Study the drawing (mm; zero at the part's minimum x, y, z) and answer. A direction names the side the tool comes from. Coordinates: 2 decimals unless noted, no trailing zeros. Order: outer loops, then holes, each group sorted by start corner. A loop starts at its lowest first (then second) coordinate and runs counter-clockwise, first axis right, second up.
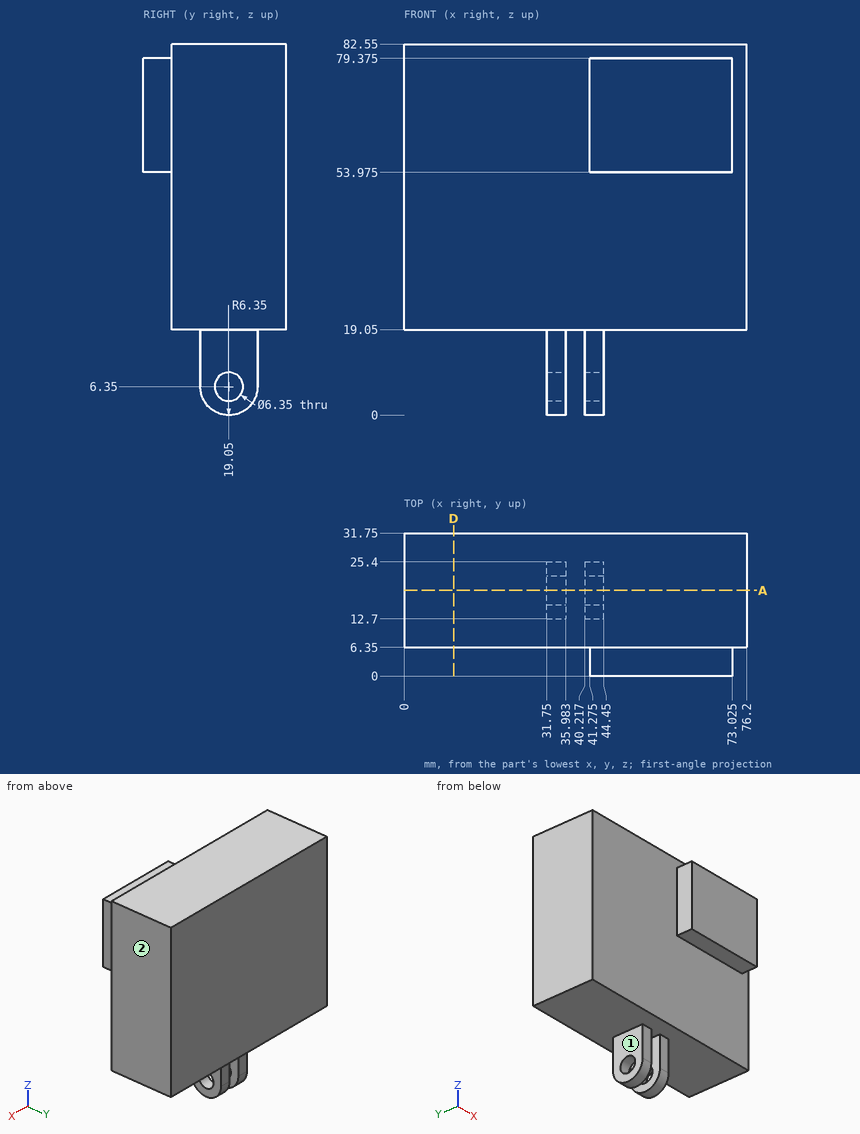
(1) Find section D-D (x = 11). Write down the section's boundary in (y, z).
(2) Each of these flat-tipped pins is pushed along its axis until it touches: pin 1 Ø8.5 at (y, z) = (19.05, 6.35) entering from +X; pin 2 Ø14 at (y, z) = (17, 6) entering from -X; pin 3 Ø3.5 at (x, z) = (33, 14) entering from +Y. Where does it stop, or does it pass through?
(3) Consider line 1 (Y direction, x = 41, z = 6) (1 decimal); line 2 (Y direction, x = 16.5, z = 30); line 3 (Z direction, x = 11.5, y = 11). Determine where each line is inside the solid, lowest interval first.
(4) Find section A-A (y = 19.05). Give the number of separate pieces and of enclosed holes in the cut face, and give its area (3 significant figures).
(5) For the marked faces 1 and 2, determine the directions among +Z, -Z, +X, -X, +Y, -Y from which every point of the face is accessible in a straight line to the end or side of a thin tool.
Findings below:
1. outline: (6.35, 19.05) - (31.75, 19.05) - (31.75, 82.55) - (6.35, 82.55) - close
2. pin 1: stops at x = 44.45
2. pin 2: stops at x = 31.75
2. pin 3: stops at y = 25.4
3. line 1: y = 12.7 to 15.9, 22.2 to 25.4
3. line 2: y = 6.35 to 31.75
3. line 3: z = 19.05 to 82.55
4. separate pieces: 3
4. enclosed holes: 0
4. area: 4,950 mm2
5. face 1: -Z, -X, +Y, -Y
5. face 2: +Z, -Z, +X, +Y, -Y
